For this review, take the finished solid that the model builds, in its own axes (mm). A direction names the side the tool comes from. Round coordinates to 2 decimals unless told otherwise and drop trailing zeros. Write each loop counter-clockwise with the first axis right and the second up, starting at its lowest first coordinate (ties: lowest second). Pieces come first, ordered by that corner, then holes. Notation, with made-up numbers: (86.5, 33) - (116.5, 33) arc R15 ccw to (116.5, 54) - close; hole circle Ø11 at (16.5, -35.75). An arc over 180 degrees is marked (long way). Answer in a Markdown table with one row per item. Add a question column.
Autodesk Inventor part; units mm, degrees
ref_plane "YZ Plane" through (0, 0, 0) normal (1, 0, 0) x (0, 1, 0)
ref_plane "XZ Plane" through (0, 0, 0) normal (0, 1, 0) x (-1, 0, 0)
ref_plane "XY Plane" through (0, 0, 0) normal (0, 0, 1) x (1, 0, 0)
sketch "Sketch1" plane through (0, 0, 0) normal (0, 0, 1) x (1, 0, 0)
  line L0 (0, 0) -> (50.8, 0)
  line L1 (50.8, 0) -> (50.8, 88.9)
  line L2 (50.8, 88.9) -> (0, 88.9)
  line L3 (0, 88.9) -> (0, 0)
  dimension "d0" = 50.8
  dimension "d1" = 88.9
extrude "Extrusion1" add sketch "Sketch1" along normal blind 25.4
shell "Shell1" thickness 3.175 removed faces 2 at (33.8667, 88.9, 8.4667) at (16.9333, 0, 16.9333)
sketch "Sketch2" plane through (0, 0, 25.4) normal (0, 0, 1) x (1, 0, 0)
  line L0 (0, 0) -> (0, 88.9)
  line L1 (50.8, 0) -> (0, 0)
  line L2 (50.8, 88.9) -> (50.8, 0)
  line L3 (12.7, 63.5) -> (38.1, 63.5) construction
  line L4 (38.1, 63.5) -> (38.1, 12.7) construction
  line L5 (38.1, 12.7) -> (12.7, 12.7) construction
  line L6 (12.7, 12.7) -> (12.7, 63.5) construction
  line L7 (12.7, 63.5) -> (0, 63.5) construction
  line L8 (38.1, 63.5) -> (50.8, 63.5) construction
  line L9 (38.1, 12.7) -> (38.1, 0) construction
  circle A0 centre (12.7, 12.7) radius 2.4384
  circle A1 centre (38.1, 12.7) radius 2.4384
  circle A2 centre (38.1, 63.5) radius 2.4384
  circle A3 centre (12.7, 63.5) radius 2.4384
  dimension "d5" = 50.8
  dimension "d6" = 25.4
  dimension "d7" = 12.7
  dimension "d8" = 4.8768
extrude "Extrusion2" cut sketch "Sketch2" against normal up to next
sketch "Sketch3" plane through (50.8, 0, 0) normal (1, 0, 0) x (0, 0, -1)
  line L0 (0, 0) -> (-25.4, 0)
  line L1 (0, 0) -> (0, 88.9)
  line L2 (-22.225, 0) -> (0, 22.225)
  line L3 (0, 22.225) -> (0, 0)
  line L4 (0, 0) -> (-22.225, 0)
  dimension "d11" = 22.225
  dimension "d12" = 22.225
extrude "Extrusion3" cut sketch "Sketch3" against normal through all
sketch "Sketch5" plane through (0, 0, 0) normal (0, 0, -1) x (-1, 0, 0)
  line L0 (0, 88.9) -> (0, 22.225)
  circle A0 centre (-25.4, 63.5) radius 14.2875
  point P0 (0, 0)
  dimension "d19" = 63.5
  dimension "d20" = 28.575
  dimension "d21" = 25.4
extrude "Extrusion5" cut sketch "Sketch5" against normal up to next
properties part number "BearingMount" material "Aluminum-6061"
Q1. Add section A-A on x = 25.4. Count the separate pieces of the cut face and the enclosed holes in it, then the cut area to 3 significant figures.
Q2. To check wall thickness, follow probe 1 along Z at (x, y) = (7, 37.5) (3 decimals); probe 2 along X at (y, z) = (70.5, 21.25) (3 decimals); probe 3 along Z at (x, y) = (26, 13) (3 decimals). State the ranges of each line that lie inside material, in increasing order.
Q3. Add section B-B on y = 63.5. State the section outline as (x, z) points (1 decimal), then the cut area to 3 significant figures.
Q4. Add section C-C on z = 8. State the section outline as (x, y) points (3 decimals), then the cut area to 3 significant figures.
Q5. Tool access review of faces 1 (the face through (27.26, 77.666, 1.565)), 2 (the face through (26, 88.9, 2)), 3 (the face through (39.23, 61.34, 23.83)), 4 (the face through (3.175, 45, 13)): name each direction out of +Z, -Z, +X, -X, +Y, -Y from which nothing blocks a thin tool from reaching the whole face with its end or side.
Q6. Draft analysis for pull direction X (two halves, no side actions). For faces 5 (the face through (50.8, 44, 13)), 6 (the face through (25, 49, 0)), 7 (the face through (13.83, 10.54, 23.83)), state which applies: released by +X, released by -X, zero draft, split by the parting line, or undercut.
Q7. Add section D-D on x = 44. State the section outline as (y, z) points (3 decimals), then the cut area to 3 significant figures.
Answer sheet:
| question | item | result |
|---|---|---|
| 1 | separate pieces | 3 |
| 1 | enclosed holes | 0 |
| 1 | area | 408 mm² |
| 2 | probe 1 | z = 0 to 3.175, 22.225 to 25.4 |
| 2 | probe 2 | x = 0 to 3.175, 47.625 to 50.8 |
| 2 | probe 3 | z = 22.225 to 25.4 |
| 3 | outline | (0, 0) - (11.1, 0) - (11.1, 3.2) - (3.2, 3.2) - (3.2, 22.2) - (10.3, 22.2) - (10.3, 25.4) - (0, 25.4) - close; (15.1, 22.2) - (35.7, 22.2) - (35.7, 25.4) - (15.1, 25.4) - close; (39.7, 0) - (50.8, 0) - (50.8, 25.4) - (40.5, 25.4) - (40.5, 22.2) - (47.6, 22.2) - (47.6, 3.2) - (39.7, 3.2) - close |
| 3 | area | 322 mm² |
| 4 | outline | (0, 14.225) - (3.175, 14.225) - (3.175, 88.9) - (0, 88.9) - close; (47.625, 14.225) - (50.8, 14.225) - (50.8, 88.9) - (47.625, 88.9) - close |
| 4 | area | 474 mm² |
| 5 | face 1 | -Z |
| 5 | face 2 | +Z, -Z, +X, -X, +Y |
| 5 | face 3 | +Z |
| 5 | face 4 | +Y, -Y |
| 6 | face 5 | released by +X |
| 6 | face 6 | zero draft |
| 6 | face 7 | undercut |
| 7 | outline | (0, 22.225) - (88.9, 22.225) - (88.9, 25.4) - (0, 25.4) - close; (19.05, 3.175) - (22.225, 0) - (88.9, 0) - (88.9, 3.175) - close |
| 7 | area | 499 mm² |
